Autodesk Inventor part; units mm, degrees
ref_plane "YZ Plane" through (0, 0, 0) normal (1, 0, 0) x (0, 1, 0)
ref_plane "XZ Plane" through (0, 0, 0) normal (0, 1, 0) x (-1, 0, 0)
ref_plane "XY Plane" through (0, 0, 0) normal (0, 0, 1) x (1, 0, 0)
sketch "Sketch1" plane through (0, 0, 0) normal (0, 0, 1) x (1, 0, 0)
  line L0 (0, 0) -> (10.414, 0)
  line L1 (10.414, 0) -> (10.414, 50.8)
  line L2 (10.414, 50.8) -> (0, 50.8)
  line L3 (0, 50.8) -> (0, 0)
  dimension "d0" = 10.414
  dimension "d1" = 50.8
extrude "Extrusion1" add sketch "Sketch1" along normal blind 1.651
sketch "Sketch2" plane through (0, 0, 1.651) normal (0, 0, 1) x (1, 0, 0)
  line L0 (0, 0) -> (10.414, 0)
  line L1 (5.207, 0) -> (3.937, 0)
  line L2 (3.937, 0) -> (3.937, 3.302)
  circle A0 centre (3.937, 3.302) radius 1.778
  line L3 (10.414, 50.8) -> (0, 50.8)
  line L4 (5.207, 50.8) -> (3.937, 50.8)
  line L5 (3.937, 50.8) -> (3.937, 47.498)
  circle A1 centre (3.937, 47.498) radius 1.778
  line L6 (3.937, 47.498) -> (3.937, 41.275)
  line L7 (3.937, 41.275) -> (3.937, 35.052)
  line L8 (3.937, 35.052) -> (3.937, 28.829)
  line L9 (3.937, 28.829) -> (3.937, 22.606)
  line L10 (3.937, 22.606) -> (3.937, 16.383)
  line L11 (3.937, 16.383) -> (3.937, 10.16)
  line L12 (3.937, 10.16) -> (3.937, 3.302)
  circle A2 centre (3.937, 10.16) radius 1.778
  circle A3 centre (3.937, 16.383) radius 1.778
  circle A4 centre (3.937, 22.606) radius 1.778
  circle A5 centre (3.937, 28.829) radius 1.778
  circle A6 centre (3.937, 35.052) radius 1.778
  circle A7 centre (3.937, 41.275) radius 1.778
  line L13 (1.4605, 45.0215) -> (6.4135, 45.0215)
  line L14 (6.4135, 45.0215) -> (6.4135, 49.9745)
  line L15 (6.4135, 49.9745) -> (1.4605, 49.9745)
  line L16 (1.4605, 49.9745) -> (1.4605, 45.0215)
  line L17 (1.4605, 45.0215) -> (6.4135, 49.9745) construction
  line L18 (6.4135, 45.0215) -> (1.4605, 49.9745) construction
  line L19 (1.4605, 38.7985) -> (6.4135, 38.7985)
  line L20 (6.4135, 38.7985) -> (6.4135, 43.7515)
  line L21 (6.4135, 43.7515) -> (1.4605, 43.7515)
  line L22 (1.4605, 43.7515) -> (1.4605, 38.7985)
  line L23 (1.4605, 38.7985) -> (6.4135, 43.7515) construction
  line L24 (6.4135, 38.7985) -> (1.4605, 43.7515) construction
  line L25 (1.4605, 32.5755) -> (6.4135, 32.5755)
  line L26 (6.4135, 32.5755) -> (6.4135, 37.5285)
  line L27 (6.4135, 37.5285) -> (1.4605, 37.5285)
  line L28 (1.4605, 37.5285) -> (1.4605, 32.5755)
  line L29 (1.4605, 32.5755) -> (6.4135, 37.5285) construction
  line L30 (6.4135, 32.5755) -> (1.4605, 37.5285) construction
  line L31 (1.4605, 26.3525) -> (6.4135, 26.3525)
  line L32 (6.4135, 26.3525) -> (6.4135, 31.3055)
  line L33 (6.4135, 31.3055) -> (1.4605, 31.3055)
  line L34 (1.4605, 31.3055) -> (1.4605, 26.3525)
  line L35 (1.4605, 26.3525) -> (6.4135, 31.3055) construction
  line L36 (6.4135, 26.3525) -> (1.4605, 31.3055) construction
  line L37 (1.4605, 20.1295) -> (6.4135, 20.1295)
  line L38 (6.4135, 20.1295) -> (6.4135, 25.0825)
  line L39 (6.4135, 25.0825) -> (1.4605, 25.0825)
  line L40 (1.4605, 25.0825) -> (1.4605, 20.1295)
  line L41 (1.4605, 20.1295) -> (6.4135, 25.0825) construction
  line L42 (6.4135, 20.1295) -> (1.4605, 25.0825) construction
  line L43 (1.4605, 13.9065) -> (6.4135, 13.9065)
  line L44 (6.4135, 13.9065) -> (6.4135, 18.8595)
  line L45 (6.4135, 18.8595) -> (1.4605, 18.8595)
  line L46 (1.4605, 18.8595) -> (1.4605, 13.9065)
  line L47 (1.4605, 13.9065) -> (6.4135, 18.8595) construction
  line L48 (6.4135, 13.9065) -> (1.4605, 18.8595) construction
  line L49 (1.4605, 7.6835) -> (6.4135, 7.6835)
  line L50 (6.4135, 7.6835) -> (6.4135, 12.6365)
  line L51 (6.4135, 12.6365) -> (1.4605, 12.6365)
  line L52 (1.4605, 12.6365) -> (1.4605, 7.6835)
  line L53 (1.4605, 7.6835) -> (6.4135, 12.6365) construction
  line L54 (6.4135, 7.6835) -> (1.4605, 12.6365) construction
  line L55 (1.4605, 0.8255) -> (6.4135, 0.8255)
  line L56 (6.4135, 0.8255) -> (6.4135, 5.7785)
  line L57 (6.4135, 5.7785) -> (1.4605, 5.7785)
  line L58 (1.4605, 5.7785) -> (1.4605, 0.8255)
  line L59 (1.4605, 0.8255) -> (6.4135, 5.7785) construction
  line L60 (6.4135, 0.8255) -> (1.4605, 5.7785) construction
  dimension "d4" = 1.27
  dimension "d5" = 3.302
  dimension "d6" = 3.556
  dimension "d7" = 3.302
  dimension "d8" = 3.556
  dimension "d9" = 6.223
  dimension "d10" = 6.223
  dimension "d11" = 6.223
  dimension "d12" = 6.223
  dimension "d13" = 6.223
  dimension "d14" = 6.223
  dimension "d15" = 3.556
  dimension "d16" = 3.556
  dimension "d17" = 3.556
  dimension "d18" = 3.556
  dimension "d19" = 3.556
  dimension "d20" = 3.556
  dimension "d21" = 4.953
  dimension "d22" = 4.953
  dimension "d23" = 4.953
  dimension "d24" = 4.953
  dimension "d25" = 4.953
  dimension "d26" = 4.953
  dimension "d27" = 4.953
  dimension "d28" = 4.953
  dimension "d29" = 4.953
  dimension "d30" = 4.953
  dimension "d31" = 4.953
  dimension "d32" = 4.953
extrude "Extrusion2" add sketch "Sketch2" along normal blind 1.778 contours L55 L58 L57 L12 A0 L2 | L13 L16 L15 L5 A1 L6 | L6 A1 L5 L15 L14 L13 | L19 L22 L21 L6 A7 L7 | L7 A7 L6 L21 L20 L19 | L25 L28 L27 L7 A6 L8 | L8 A6 L7 L27 L26 L25 | L31 L34 L33 L8 A5 L9 | L9 A5 L8 L33 L32 L31 | L37 L40 L39 L9 A4 L10 | L10 A4 L9 L39 L38 L37 | L43 L46 L45 L10 A3 L11 | L11 A3 L10 L45 L44 L43 | L49 L52 L51 L11 A2 L12 | L12 A2 L11 L51 L50 L49 | L2 A0 L12 L57 L56 L55
sketch "Sketch3" plane through (0, 0, 1.651) normal (0, 0, 1) x (1, 0, 0)
  circle A0 centre (3.937, 3.302) radius 1.778
  circle A1 centre (3.937, 3.302) radius 1.778
  circle A2 centre (3.937, 10.16) radius 1.778
  circle A3 centre (3.937, 10.16) radius 1.778
  circle A4 centre (3.937, 16.383) radius 1.778
  circle A5 centre (3.937, 16.383) radius 1.778
  circle A6 centre (3.937, 22.606) radius 1.778
  circle A7 centre (3.937, 22.606) radius 1.778
  circle A8 centre (3.937, 28.829) radius 1.778
  circle A9 centre (3.937, 28.829) radius 1.778
  circle A10 centre (3.937, 35.052) radius 1.778
  circle A11 centre (3.937, 35.052) radius 1.778
  circle A12 centre (3.937, 41.275) radius 1.778
  circle A13 centre (3.937, 41.275) radius 1.778
  circle A14 centre (3.937, 47.498) radius 1.778
  circle A15 centre (3.937, 47.498) radius 1.778
  point P0 (0, 0)
extrude "Extrusion3" add sketch "Sketch3" along normal blind 1.651
sketch "Sketch4" plane through (0, 0, 1.651) normal (0, 0, 1) x (1, 0, 0)
  line L0 (1.4605, 12.6365) -> (6.4135, 12.6365)
  line L1 (6.4135, 13.9065) -> (6.4135, 18.8595)
  line L2 (6.4135, 12.6365) -> (6.4135, 13.9065)
  line L3 (6.4135, 13.9065) -> (6.4135, 13.2715)
  line L4 (10.414, 0) -> (10.414, 50.8)
  line L5 (10.414, 13.2715) -> (6.4135, 13.2715)
  circle A0 centre (8.4138, 13.2715) radius 1.3335
  line L6 (1.4605, 37.5285) -> (6.4135, 37.5285)
  line L7 (6.4135, 38.7985) -> (6.4135, 37.5285)
  line L8 (6.4135, 38.1635) -> (10.414, 38.1635)
  circle A1 centre (8.4138, 38.1635) radius 1.3335
  point P0 (0, 0)
extrude "Extrusion4" cut sketch "Sketch4" against normal blind 1.651
properties part number "Neopixel_Stick"
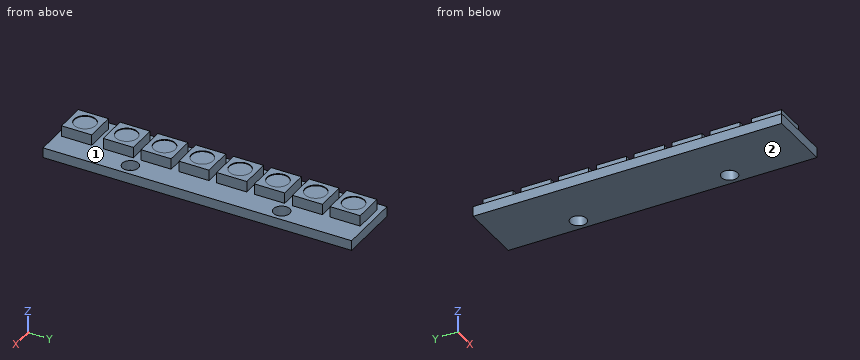
Could you check a few things on this model? Use its own coordinates, in mm. Face numbers are marked on the shaded views. Give positions to 0.01 mm unless a question says otherwise; leave off trailing zeros. Write each loop counter-clockwise with the first axis right and the second up, starting at its lowest first coordinate (ties: lowest second). Pieces come first, ordered by that corner, then holes. Notation, with made-up numbers: (2, 24) -> (57, 24) arc R29 cw to (57, 49) -> close; hole circle Ø6 at (42, 81.25). An arc over 180 degrees is marked (long way). Write each question's results on one line, items separated by ' | '.
1. I need wall thicknesses on L1, parallel to Z at x = 3.5, y = 35; L2, parallel to Z at x = 7.5, y = 24.5; L3, parallel to X at y = 5.5, z = 2.1. Which ranges of each line are inside material? Lowest first, please.
Check sheet entries:
L1: z = 0 to 3.3 | L2: z = 0 to 1.65 | L3: x = 1.46 to 6.41
2. I want a section at A-A, the plane z = 2.15. Count the separate pieces of the cut face and the enclosed holes in it, then the cut area to 3 significant figures.
Check sheet entries:
separate pieces: 8 | enclosed holes: 0 | area: 196 mm²
3. I want a section at D-D, the plane x = 0.5. Write out the boundary of the cut face in (y, z), then the cut area to 3 significant figures.
Check sheet entries:
outline: (0, 0) -> (50.8, 0) -> (50.8, 1.65) -> (0, 1.65) -> close | area: 83.9 mm²
4. If we mould it in two halves opening along Y, with no side actions, what happens to the marked faces 1 and 2? For each: released by +Y, released by -Y, zero draft, split by the parting line, or undercut.
Check sheet entries:
face 1: undercut | face 2: zero draft
5. Will these pins go through, and if not, where does the flat tip stop? pin 1 Ø0.9 at (y, z) = (34, 2.5) entering from -X; pin 2 Ø0.5 at (y, z) = (3.5, 3) entering from +X; pin 3 Ø0.5 at (x, z) = (5, 2) entering from -Y.
Check sheet entries:
pin 1: stops at x = 1.46 | pin 2: stops at x = 6.41 | pin 3: stops at y = 0.83
6. I want a section at B-B, the plane x = 8.5. Write out the boundary of the cut face in (y, z), then the cut area to 3 significant figures.
Check sheet entries:
outline: (0, 0) -> (11.94, 0) -> (11.94, 1.65) -> (0, 1.65) -> close; (14.6, 0) -> (36.83, 0) -> (36.83, 1.65) -> (14.6, 1.65) -> close; (39.49, 0) -> (50.8, 0) -> (50.8, 1.65) -> (39.49, 1.65) -> close | area: 75.1 mm²
